Build history of the part. All positions in model axes, mm. Face numbers are marked on the shaded views. A direction names the side the tool comes from. Give positions to 0.01 mm unless a question says otherwise; leave off trailing zeros. Loops run counter-clockwise (first coordinate to the right, second up) from the corner with the lowest first, then second, coordinate; pieces in that order, holes last. Notation, with made-up numbers: M 38,-39 L 42,-39 A14 cw 42,-34 Z; hole C 12.25,47.5 d3. An arc over 180 degrees is marked long. Answer as a JSON object with one key per item and string values. Group by question number.
1. Slice it at A-A (x = 0). List the corners of the cut face in (y, z) (3 decimals).
2. Drop flat-ended pins along their axis: pin 1 Ø8 at (x, z) = (32, 7) entering from -Y; pin 2 Ø3 at (y, z) = (-4.5, 17.5) entering from +X; pin 3 Ø10 at (x, y) = (-5.5, -13) entering from -Z (3 decimals); pin 4 Ø20.5 at (x, y) = (-3.5, 10) entering from -Z. Give the stop position or say it passes through.
3. Slice it at B-B (z = 15.5). Give the number of separate pieces and of enclosed holes in the cut face, then the cut area to 3 significant figures.
4. Drill centre lines: line 1 along Y through (x, z) = (0, 19.25) (3 decimals); line 2 along X through (y, z) = (4, 9.25); line 3 along Y through (x, z) = (0, 6.75) (3 decimals). Where is each one in solid material? Low to high. Write a range as [from, to].
5. Mould opens along Y. For the marked faces 3, 4, 5 and 6 say: released by +Y, released by -Y, zero draft, split by the parting line, or undercut.
6. 3-axis set-ups, long thin cutter, end or side, ignore diameter. For the marked faces 1 and 2: which of +Z, -Z, +X, -X, +Y, -Y reach the whole face in a straight line?
from build123d import *

# Parameters (mm, degrees)
SKETCH1_R          = 5.1562
EXTRUDE1_DEPTH     = 23.495
SKETCH6_R          = 20.64385
CUT_EXTRUDE1_DEPTH = 17.145
SKETCH7_R          = 15.875
CUT_EXTRUDE2_DEPTH = 7.35
FILLET1_R          = 0.127


with BuildPart() as part:
    # Sketch1 → Extrude1 (new body)
    with BuildSketch(Plane.XY):
        with BuildLine():
            Line((-39.215785714, 9.802584203), (-14.695714286, 24.506460508))
            ThreePointArc((-14.695714286, 24.506460508), (0, 28.575), (14.695714286, 24.506460508))
            Line((14.695714286, 24.506460508), (39.215785714, 9.802584203))
            ThreePointArc((39.215785714, 9.802584203), (44.7675, 0), (39.215785714, -9.802584203))
            Line((39.215785714, -9.802584203), (14.695714286, -24.506460508))
            ThreePointArc((14.695714286, -24.506460508), (0, -28.575), (-14.695714286, -24.506460508))
            Line((-14.695714286, -24.506460508), (-39.215785714, -9.802584203))
            ThreePointArc((-39.215785714, -9.802584203), (-44.7675, 0), (-39.215785714, 9.802584203))
        make_face()
        with Locations((-33.3375, 0)):
            Circle(SKETCH1_R, mode=Mode.SUBTRACT)
        with Locations((33.3375, 0)):
            Circle(SKETCH1_R, mode=Mode.SUBTRACT)
    extrude(amount=EXTRUDE1_DEPTH)

    # Sketch6 → Cut-Extrude1 (cut)
    with BuildSketch(Plane.XY):
        Circle(SKETCH6_R)
    extrude(amount=CUT_EXTRUDE1_DEPTH, mode=Mode.SUBTRACT)

    # Sketch7 → Cut-Extrude2 (cut, through all)
    with BuildSketch(Plane(origin=(0, 0, 17.145), x_dir=(-1, 0, 0), z_dir=(0, 0, -1))):
        Circle(SKETCH7_R)
    extrude(amount=-CUT_EXTRUDE2_DEPTH, mode=Mode.SUBTRACT)

    # Fillet1
    fillet1_edges = [part.edges().sort_by_distance(p)[0] for p in [
        (-20.64385, 0, 17.145),
    ]]
    fillet(fillet1_edges, radius=FILLET1_R)


solid = part.part
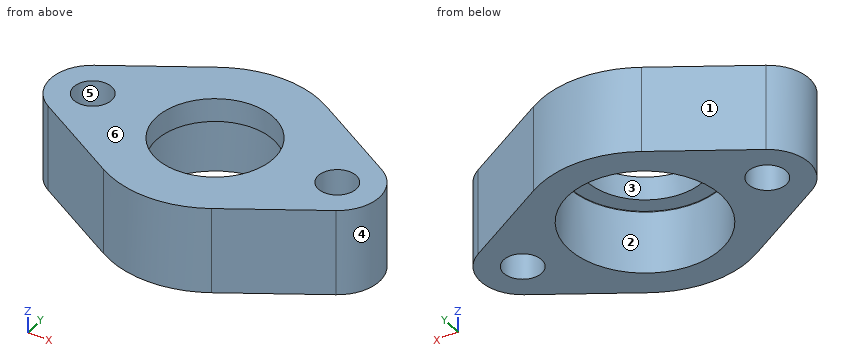
Established:
{
 "1": {"outline": "M -28.575,0 L -20.644,0 L -20.644,17.018 A0.127 cw -20.517,17.145 L -15.875,17.145 L -15.875,23.495 L -28.575,23.495 Z; M 15.875,17.145 L 20.517,17.145 A0.127 cw 20.644,17.018 L 20.644,0 L 28.575,0 L 28.575,23.495 L 15.875,23.495 Z"},
 "2": {"pin 1": "stops at y = -16.53", "pin 2": "stops at x = 44.37", "pin 3": "stops at z = 17.145", "pin 4": "stops at z = 0"},
 "3": {"separate pieces": "1", "enclosed holes": "3", "area": "1,930 mm^2"},
 "4": {"line 1": "y = [-28.575, -15.875], [15.875, 28.575]", "line 2": "x = [-44.04, -36.59], [-30.08, -20.25], [20.25, 30.08], [36.59, 44.04]", "line 3": "y = [-28.575, -20.644], [20.644, 28.575]"},
 "5": {"face 3": "undercut", "face 4": "split by the parting line", "face 5": "undercut", "face 6": "zero draft"},
 "6": {"face 1": "+Z, -Z, -X, +Y", "face 2": "-Z"}
}
